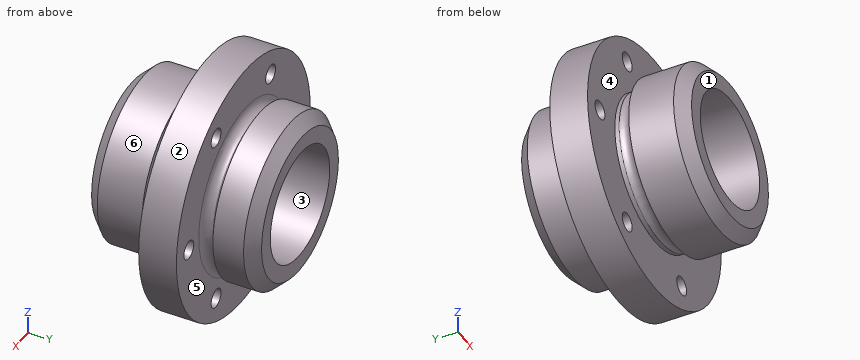
from build123d import *

# Parameters (mm, degrees)
CHAMFER2_SIZE      = 5
FILLET1_R          = 4
CUT_EXTRUDE1_REACH = 92.2
SKETCH2_R          = 4


with BuildPart() as part:
    # Sketch1 → Revolve1 (revolve)
    with BuildSketch(Plane.XY, mode=Mode.PRIVATE) as revolve1_sk:
        with BuildLine():
            ThreePointArc((-36, -12.335343788), (-31.975370241, -10.570389375), (-32, -6.175835683))
            Line((-32, -6.175835683), (-32, -4.335343788))
            Line((-32, -4.335343788), (-54, -4.335343788))
            Line((-54, -4.335343788), (-54, 11.664656212))
            Line((-54, 11.664656212), (-32, 11.664656212))
            Line((-32, 11.664656212), (-32, 17.664656212))
            Line((-32, 17.664656212), (-36, 17.664656212))
            Line((-36, 17.664656212), (-36, 35.664656212))
            Line((-36, 35.664656212), (-24, 35.664656212))
            Line((-24, 35.664656212), (-24, -36.335343788))
            Line((-24, -36.335343788), (-36, -36.335343788))
            Line((-36, -36.335343788), (-36, -12.335343788))
        make_face()
    revolve(revolve1_sk.sketch.rotate(Axis((0, 0, 0), (0, 1, 0)), 270), axis=Axis((0, 0, 0), (0, 1, 0)))

    # Chamfer2
    chamfer2_edges = [part.edges().sort_by_distance(p)[0] for p in [
        (0, 35.664656212, 36),
        (0, -36.335343788, 36),
    ]]
    chamfer(chamfer2_edges, length=CHAMFER2_SIZE)

    # Fillet1
    fillet1_edges = [part.edges().sort_by_distance(p)[0] for p in [
        (0, 11.664656212, 32),
    ]]
    fillet(fillet1_edges, radius=FILLET1_R)

    # Sketch2 → Cut-Extrude1 (cut, up to next)
    with BuildSketch(Plane(origin=(0, 11.664656212, 0), x_dir=(1, 0, 0), z_dir=(0, 1, 0)), mode=Mode.PRIVATE) as cut_extrude1_sk1:
        with Locations(Location((44, 0, 0), (0, 0, 270))):
            Circle(SKETCH2_R)
    cut_extrude1_tool1 = extrude(cut_extrude1_sk1.sketch, amount=-CUT_EXTRUDE1_REACH, mode=Mode.PRIVATE) & part.part
    # Sketch2 → Cut-Extrude1 (cut, up to next)
    with BuildSketch(Plane(origin=(0, 11.664656212, 0), x_dir=(1, 0, 0), z_dir=(0, 1, 0)), mode=Mode.PRIVATE) as cut_extrude1_sk2:
        with Locations(Location((22, -38.105117767, 0), (0, 0, 270))):
            Circle(SKETCH2_R)
    cut_extrude1_tool2 = extrude(cut_extrude1_sk2.sketch, amount=-CUT_EXTRUDE1_REACH, mode=Mode.PRIVATE) & part.part
    # Sketch2 → Cut-Extrude1 (cut, up to next)
    with BuildSketch(Plane(origin=(0, 11.664656212, 0), x_dir=(1, 0, 0), z_dir=(0, 1, 0)), mode=Mode.PRIVATE) as cut_extrude1_sk3:
        with Locations(Location((-22, -38.105117767, 0), (0, 0, 270))):
            Circle(SKETCH2_R)
    cut_extrude1_tool3 = extrude(cut_extrude1_sk3.sketch, amount=-CUT_EXTRUDE1_REACH, mode=Mode.PRIVATE) & part.part
    # Sketch2 → Cut-Extrude1 (cut, up to next)
    with BuildSketch(Plane(origin=(0, 11.664656212, 0), x_dir=(1, 0, 0), z_dir=(0, 1, 0)), mode=Mode.PRIVATE) as cut_extrude1_sk4:
        with Locations(Location((-44, 0, 0), (0, 0, 270))):
            Circle(SKETCH2_R)
    cut_extrude1_tool4 = extrude(cut_extrude1_sk4.sketch, amount=-CUT_EXTRUDE1_REACH, mode=Mode.PRIVATE) & part.part
    # Sketch2 → Cut-Extrude1 (cut, up to next)
    with BuildSketch(Plane(origin=(0, 11.664656212, 0), x_dir=(1, 0, 0), z_dir=(0, 1, 0)), mode=Mode.PRIVATE) as cut_extrude1_sk5:
        with Locations(Location((-22, 38.105117767, 0), (0, 0, 270))):
            Circle(SKETCH2_R)
    cut_extrude1_tool5 = extrude(cut_extrude1_sk5.sketch, amount=-CUT_EXTRUDE1_REACH, mode=Mode.PRIVATE) & part.part
    # Sketch2 → Cut-Extrude1 (cut, up to next)
    with BuildSketch(Plane(origin=(0, 11.664656212, 0), x_dir=(1, 0, 0), z_dir=(0, 1, 0)), mode=Mode.PRIVATE) as cut_extrude1_sk6:
        with Locations(Location((22, 38.105117767, 0), (0, 0, 270))):
            Circle(SKETCH2_R)
    cut_extrude1_tool6 = extrude(cut_extrude1_sk6.sketch, amount=-CUT_EXTRUDE1_REACH, mode=Mode.PRIVATE) & part.part
    add(cut_extrude1_tool1.solids().sort_by_distance((44, 11.664656, 0))[0], mode=Mode.SUBTRACT)
    add(cut_extrude1_tool2.solids().sort_by_distance((22, 11.664656, 38.105118))[0], mode=Mode.SUBTRACT)
    add(cut_extrude1_tool3.solids().sort_by_distance((-22, 11.664656, 38.105118))[0], mode=Mode.SUBTRACT)
    add(cut_extrude1_tool4.solids().sort_by_distance((-44, 11.664656, 0))[0], mode=Mode.SUBTRACT)
    add(cut_extrude1_tool5.solids().sort_by_distance((-22, 11.664656, -38.105118))[0], mode=Mode.SUBTRACT)
    add(cut_extrude1_tool6.solids().sort_by_distance((22, 11.664656, -38.105118))[0], mode=Mode.SUBTRACT)


solid = part.part
CAD build for the part. Positions are in the model's coordinates, mm. Face numbers are marked on the shaded views. A direction names the side the tool comes from. Give positions to 0.01 mm unless a question says otherwise; leave off trailing zeros. Write each loop counter-clockwise with the first axis right and the second up, starting at its lowest first coordinate (ties: lowest second). Pieces come first, ordered by that corner, then holes. Notation, with made-up numbers: (-37, -39.75) -> (-30, -39.75) arc R23 ccw to (-30, -0.75) -> close; hole circle Ø8 at (55, -2). An arc over 180 degrees is marked (long way). Return JSON: item names as keys, results as strings.
Item 1: Band-saw the part on A-A (y = 7.5). List the corners of the cut face in (x, z).
Answer below:
{"outline": "circle Ø108 at (0, 0); hole circle Ø8 at (-44, 0); hole circle Ø8 at (-22, -38.11); hole circle Ø8 at (-22, 38.11); hole circle Ø48 at (0, 0); hole circle Ø8 at (22, -38.11); hole circle Ø8 at (22, 38.11); hole circle Ø8 at (44, 0)"}
Item 2: Two-plate mould, pull along Z, no slides. Class the marked faces 1, 2 and 3: +Z half, -Z half, draft (parallel to the pull), parting line (faces both ways), or undercut.
Answer below:
{"face 1": "draft", "face 2": "parting line", "face 3": "undercut"}
Item 3: Band-saw the part on C-C (z = 0). Give the number of separate pieces and of enclosed holes in the cut face, then the cut area to 3 significant figures.
Answer below:
{"separate pieces": "4", "enclosed holes": "0", "area": "1,890 mm2"}
Item 4: Band-saw the part on B-B (x = 44). List the corners of the cut face in (y, z), then the cut area to 3 significant figures.
Answer below:
{"outline": "(-4.34, -31.3) -> (11.66, -31.3) -> (11.66, -4) -> (-4.34, -4) -> close; (-4.34, 4) -> (11.66, 4) -> (11.66, 31.3) -> (-4.34, 31.3) -> close", "area": "874 mm2"}
Item 5: Tool access for the marked faces 4, 5 and 6: list every direction of +Z, -Z, +X, -X, +Y, -Y with a clear straight run to the whole face (end or side of a thin tool).
Answer below:
{"face 4": "none", "face 5": "+Y", "face 6": "-Y"}
Item 6: Band-saw the part on D-D (y = -25). List the corners of the cut face in (x, z).
Answer below:
{"outline": "circle Ø72 at (0, 0); hole circle Ø48 at (0, 0)"}
Item 7: Drop flat-ended pins along their axis: pin 1 (9 mm diameter, centred on x = -44, z = 0, fed in from +Y); pin 2 (1 mm diameter, centred on x = -11.5, z = -35.5, fed in from -Y); pin 3 (7 mm diameter, centred on x = -22, z = -38.11, fed in from -Y); pin 4 (1 mm diameter, centred on y = -13.5, z = -30.5, fed in from -X). Give the stop position or say it passes through.
Answer below:
{"pin 1": "stops at y = 11.66", "pin 2": "stops at y = -4.34", "pin 3": "passes through", "pin 4": "stops at x = -19.9"}
Item 8: Drill centre lines: probe 1 along Y at (x, z) = (-35, -24); probe 2 along Z at (x, y) = (-13.5, 19); probe 3 along X at (y, z) = (-17, 10). Where is each one in solid material? Low to high.
Answer below:
{"probe 1": "y = -4.34 to 11.66", "probe 2": "z = -33.37 to -19.84, 19.84 to 33.37", "probe 3": "x = -34.58 to -21.82, 21.82 to 34.58"}
